Geometry check sheet. Reference: the model listing, model coordinates, mm. Face numbers are marked on the shaded views. Round coordinates to 2 decimals unless told otherwise and drop trailing zeros. Order: outer loops, then holes, each group sorted by start corner. A loop starts at its lowest first (then second) coordinate and runs counter-clockwise, first axis right, second up.
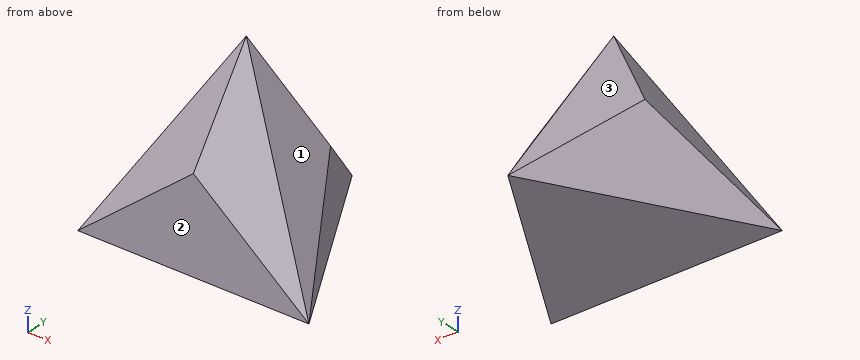
```python
from build123d import *

# Parameters (mm, degrees)
F1_DEPTH = 81.6496580928
F5_DEPTH = 100
F6_DEPTH = 100
F7_DEPTH = 100


with BuildPart() as f1:
    # F0 (on Top) → F1 (new body)
    with BuildSketch(Plane.XY):
        Polygon((-25, 0), (25, 0), (0, 43.3012701892), align=None)
        Polygon((-25, 0), (0, -43.3012701892), (25, 0), align=None)
        Polygon((-50, -43.3012701892), (0, -43.3012701892), (-25, 0), align=None)
        Polygon((0, -43.3012701892), (50, -43.3012701892), (25, 0), align=None)
    extrude(amount=F1_DEPTH)

    # F4 (on face) → F5 (cut)
    with BuildSketch(Plane(origin=(-18.75, 10.8253175473, 0), x_dir=(-0.5, -0.8660254038, 0), z_dir=(-0.8660254038, 0.5, 0))):
        Polygon((-37.5, 81.6496580928), (-37.5, 0), (12.5, 81.6496580928), align=None)
        Polygon((62.5, 81.6496580928), (12.5, 81.6496580928), (62.5, 0), align=None)
    extrude(amount=-F5_DEPTH, mode=Mode.SUBTRACT)

    # F2 (on face) → F6 (cut)
    with BuildSketch(Plane.XZ.offset(43.3012701892)):
        Polygon((-50, 81.6496580928), (-50, 0), (0, 81.6496580928), align=None)
        Polygon((50, 81.6496580928), (0, 81.6496580928), (50, 0), align=None)
    extrude(amount=-F6_DEPTH, mode=Mode.SUBTRACT)

    # F3 (on face) → F7 (cut)
    with BuildSketch(Plane(origin=(18.75, 10.8253175473, 0), x_dir=(-0.5, 0.8660254038, 0), z_dir=(0.8660254038, 0.5, 0))):
        Polygon((-62.5, 81.6496580928), (-62.5, 0), (-12.5, 81.6496580928), align=None)
        Polygon((37.5, 81.6496580928), (-12.5, 81.6496580928), (37.5, 0), align=None)
    extrude(amount=-F7_DEPTH, mode=Mode.SUBTRACT)


solid = f1.part
```
(1) Sectioned sample at A-A, the plane y = -7. Record the cut outline in (x, z), and give its area (3 significant figures).
Returned:
outline: (-29.04, 0) - (29.04, 0) - (29.04, 34.23) - (12.88, 60.62) - (0, 71.14) - (-12.88, 60.62) - (-29.04, 34.23) - close
area: 3,230 mm2
(2) Material ranges on line 1 (Z direction, x = 6.5, y = 27.5); line 2 (X direction, y = 24.5, z = 17.5); line 3 (Z direction, x = 30, y = -9.5), recorded low to high.
Returned:
line 1: z = 0 to 17.04
line 2: x = -10.85 to 10.85
line 3: z = 0 to 32.66
(3) Sectioned sample at B-B, the plane z = 5.5. Record the cut outline in (x, y).
Returned:
outline: (-46.63, -41.36) - (-43.26, -43.3) - (43.26, -43.3) - (46.63, -41.36) - (46.63, -37.47) - (3.37, 37.47) - (0, 39.41) - (-3.37, 37.47) - (-46.63, -37.47) - close
(4) Sectioned sample at C-C, the plane x = 8. Record the cut outline in (y, z).
Returned:
outline: (-43.3, 0) - (29.44, 0) - (29.44, 13.06) - (-9.81, 68.59) - (-19.05, 68.59) - (-43.3, 34.29) - close
(5) Sectioned sample at D-D, the plane y = -35. Record the cut outline in (x, z), and give its area (3 significant figures).
Returned:
outline: (-45.21, 0) - (45.21, 0) - (45.21, 7.83) - (35.62, 23.48) - (0, 52.56) - (-35.62, 23.48) - (-45.21, 7.83) - close
area: 3,010 mm2
(6) Depth check by flat-ended pin: P1, Ø5, axis at x = 28, y = -3, coming from the -Z side; P2, Ø2, axis at y = -13.5, z = 52.5, coming from the +X side; P3, Ø2, axis at x = -26, z = 35, coming from the +Y side; P4, Ø8, axis at x = 31, z = 45.5, coming from the -Y side. Enter the tip coordinate at first touch or a pass-through.
Returned:
P1: stops at z = 0
P2: stops at x = 18.46
P3: stops at y = 0
P4: passes through
(7) Draft check along X on the marked faces 1, 2 and 3. Enter one of: released by +X, released by -X, zero draft, split by the parting line, or undercut.
Returned:
face 1: released by +X
face 2: zero draft
face 3: released by -X
